The figure shows three views and two pictorial views of one solid part (mm, origin at its lowest corner). Answer the questions. A direction names the side the tool comes from. Give positions to 0.01 mm unless a question says otherwise; leave off trailing zeros. Loops run counter-clockwise (first coordinate to the right, second up) from the corner with the lowest first, then second, coordinate; pieces in that order, holes last.
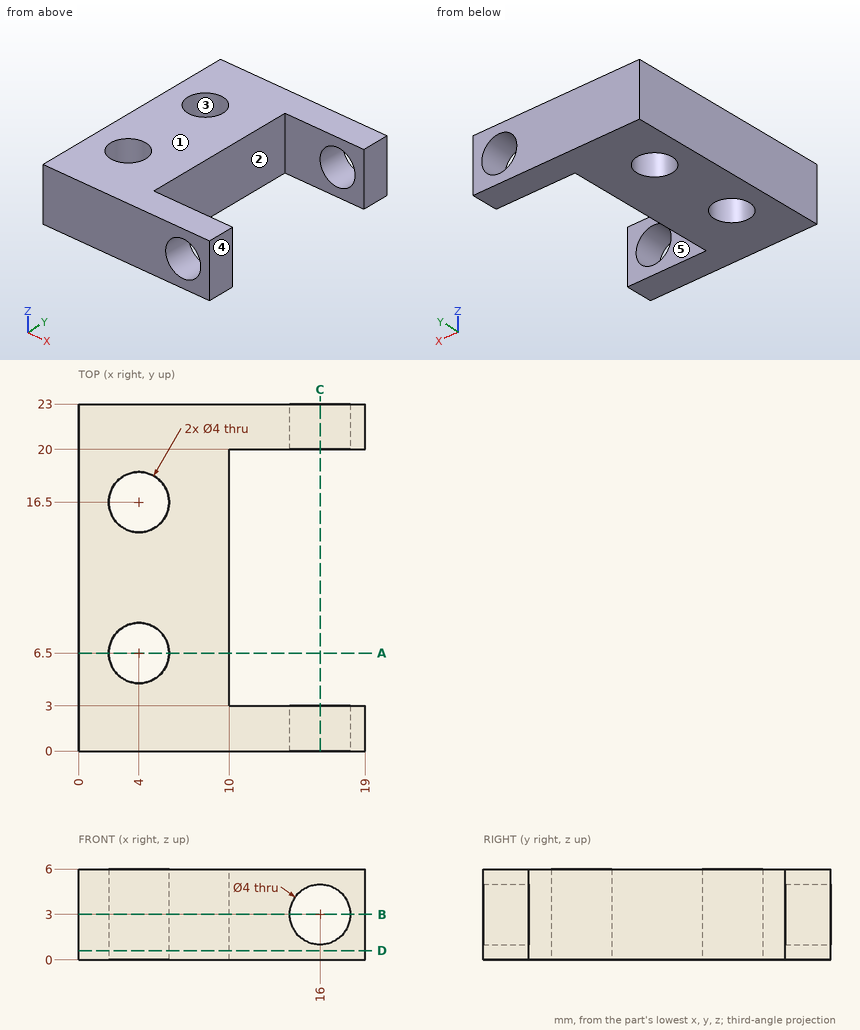
Q1. Determine the mould class of the marked faces 3, 4 and 5 for opening direction X: +X half, -X half, draft (parallel to the pull), parting line (faces both ways), or undercut.
Q2. Section B-B on z = 3 is taken. Give the vertices of the cut face in (x, y), plus the area to 3 significant figures.
Q3. Section C-C on x = 16 is taken. Give the vertices of the cut face in (y, z), plus the area to 3 significant figures.
Q4. Section A-A on y = 6.5 is taken. Give the vertices of the cut face in (x, z), plus the area to 3 significant figures.
Q5. Which of the six approach directions +Z, -Z, +X, -X, +Y, -Y give full straight-line access (tool end or side, diameter ignored) to the marked faces 1 and 2?
Q6. Given pin 1 (3 mm diameter, centred on y = 10, z = 3.5, fed in from +X), flat-ended and moving along its own axis, determine where the tip first touches the part or whether it passes through.
Q7. Section D-D on z = 0.6 is taken. Give the vertices of the cut face in (x, y).
Q8. Consider line 1 along Y through (x, z) = (10.5, 5.55); line 2 along X through (y, z) = (16.5, 4.7); line 3 along Y through (x, z) = (3.75, 1.25). Determine where each line is inside the solid, lowest interval first.
Check result:
1. face 3: undercut
1. face 4: +X half
1. face 5: draft
2. outline: (0, 0) - (14, 0) - (14, 3) - (10, 3) - (10, 20) - (14, 20) - (14, 23) - (0, 23) - close; (18, 0) - (19, 0) - (19, 3) - (18, 3) - close; (18, 20) - (19, 20) - (19, 23) - (18, 23) - close; hole circle Ø4 at (4, 6.5); hole circle Ø4 at (4, 16.5)
2. area: 235 mm2
3. outline: (0, 0) - (3, 0) - (3, 1) - (0, 1) - close; (0, 5) - (3, 5) - (3, 6) - (0, 6) - close; (20, 0) - (23, 0) - (23, 1) - (20, 1) - close; (20, 5) - (23, 5) - (23, 6) - (20, 6) - close
3. area: 12.0 mm2
4. outline: (0, 0) - (2, 0) - (2, 6) - (0, 6) - close; (6, 0) - (10, 0) - (10, 6) - (6, 6) - close
4. area: 36.0 mm2
5. face 1: +Z, +X, -X, +Y, -Y
5. face 2: +Z, -Z, +X
6. pin 1: stops at x = 10
7. outline: (0, 0) - (19, 0) - (19, 3) - (10, 3) - (10, 20) - (19, 20) - (19, 23) - (0, 23) - close; hole circle Ø4 at (4, 6.5); hole circle Ø4 at (4, 16.5)
8. line 1: y = 0 to 3, 20 to 23
8. line 2: x = 0 to 2, 6 to 10
8. line 3: y = 0 to 4.52, 8.48 to 14.52, 18.48 to 23
